Work out the finished part from the listing and answer in its coordinate system (mm). A direction names the side the tool comes from. Coordinates: 2 decimals unless noted, no trailing zeros. Order: outer loops, then holes, each group sorted by start corner. A loop starts at its lowest first (then second) coordinate and runs counter-clockwise, first axis right, second up.
```python
from build123d import *

# Parameters (mm, degrees)
F0_W      = 120.65
F0_H      = 120.65
F1_DEPTH  = 6.35
F2_W      = 12.7
F2_H      = 6.35
F3_DEPTH  = 6.351
F4_W      = 12.7
F4_H      = 6.35
F5_DEPTH  = 6.351
F6_W      = 6.35
F6_H      = 6.35
F7_DEPTH  = 6.351
F8_W      = 12.7
F8_H      = 6.35
F9_DEPTH  = 6.351
F10_W     = 12.7
F10_H     = 6.35
F11_DEPTH = 6.351
F12_W     = 6.35
F12_H     = 12.7
F13_DEPTH = 6.351
F14_W     = 6.35
F14_H     = 12.7
F15_DEPTH = 6.351
F16_W     = 6.35
F16_H     = 12.7
F17_DEPTH = 6.351
F18_W     = 12.7
F18_H     = 6.35
F19_DEPTH = 6.351
F20_W     = 12.7
F20_H     = 6.35
F20_W_2   = 6.35
F21_DEPTH = 6.351
F22_W     = 6.35
F22_H     = 12.7
F23_DEPTH = 6.351
F24_W     = 6.35
F24_H     = 12.7
F25_DEPTH = 6.351


with BuildPart() as f1:
    # F0 (on Right) → F1 (new body)
    with BuildSketch(Plane.YZ):
        Rectangle(F0_W, F0_H)
    extrude(amount=F1_DEPTH)

    # F2 (on face) → F3 (cut, through all)
    with BuildSketch(Plane(origin=(0, 0, 0), x_dir=(0, -1, 0), z_dir=(-1, 0, 0))):
        with Locations((53.975, 57.15)):
            Rectangle(F2_W, F2_H)
    extrude(amount=-F3_DEPTH, mode=Mode.SUBTRACT)

    # F4 (on face) → F5 (cut, through all)
    with BuildSketch(Plane(origin=(0, 0, 0), x_dir=(0, -1, 0), z_dir=(-1, 0, 0))):
        with Locations((28.575, 57.15)):
            Rectangle(F4_W, F4_H)
    extrude(amount=-F5_DEPTH, mode=Mode.SUBTRACT)

    # F6 (on face) → F7 (cut, through all)
    with BuildSketch(Plane(origin=(0, 0, 0), x_dir=(0, -1, 0), z_dir=(-1, 0, 0))):
        with Locations((0, 57.15)):
            Rectangle(F6_W, F6_H)
    extrude(amount=-F7_DEPTH, mode=Mode.SUBTRACT)

    # F8 (on face) → F9 (cut, through all)
    with BuildSketch(Plane(origin=(0, 0, 0), x_dir=(0, -1, 0), z_dir=(-1, 0, 0))):
        with Locations((-53.975, 57.15)):
            Rectangle(F8_W, F8_H)
    extrude(amount=-F9_DEPTH, mode=Mode.SUBTRACT)

    # F10 (on face) → F11 (cut, through all)
    with BuildSketch(Plane(origin=(0, 0, 0), x_dir=(0, -1, 0), z_dir=(-1, 0, 0))):
        with Locations((-28.575, 57.15)):
            Rectangle(F10_W, F10_H)
    extrude(amount=-F11_DEPTH, mode=Mode.SUBTRACT)

    # F12 (on face) → F13 (cut, through all)
    with BuildSketch(Plane(origin=(0, 0, 0), x_dir=(0, -1, 0), z_dir=(-1, 0, 0))):
        with Locations((-57.15, 34.925)):
            Rectangle(F12_W, F12_H)
    extrude(amount=-F13_DEPTH, mode=Mode.SUBTRACT)

    # F14 (on face) → F15 (cut, through all)
    with BuildSketch(Plane(origin=(0, 0, 0), x_dir=(0, -1, 0), z_dir=(-1, 0, 0))):
        with Locations((-57.15, 4.7625)):
            Rectangle(F14_W, F14_H)
    extrude(amount=-F15_DEPTH, mode=Mode.SUBTRACT)

    # F16 (on face) → F17 (cut, through all)
    with BuildSketch(Plane(origin=(0, 0, 0), x_dir=(0, -1, 0), z_dir=(-1, 0, 0))):
        with Locations((-57.15, -25.4)):
            Rectangle(F16_W, F16_H)
    extrude(amount=-F17_DEPTH, mode=Mode.SUBTRACT)

    # F18 (on face) → F19 (cut, through all)
    with BuildSketch(Plane(origin=(0, 0, 0), x_dir=(0, -1, 0), z_dir=(-1, 0, 0))):
        with Locations((-53.975, -57.15)):
            Rectangle(F18_W, F18_H)
        with Locations((53.975, -57.15)):
            Rectangle(F18_W, F18_H)
    extrude(amount=-F19_DEPTH, mode=Mode.SUBTRACT)

    # F20 (on face) → F21 (cut, through all)
    with BuildSketch(Plane(origin=(0, 0, 0), x_dir=(0, -1, 0), z_dir=(-1, 0, 0))):
        with Locations((-28.575, -57.15)):
            Rectangle(F20_W, F20_H)
        with Locations((0, -57.15)):
            Rectangle(F20_W_2, F20_H)
        with Locations((28.575, -57.15)):
            Rectangle(F20_W, F20_H)
    extrude(amount=-F21_DEPTH, mode=Mode.SUBTRACT)

    # F22 (on face) → F23 (cut, through all)
    with BuildSketch(Plane(origin=(0, 0, 0), x_dir=(0, -1, 0), z_dir=(-1, 0, 0))):
        with Locations((57.15, 34.925)):
            Rectangle(F22_W, F22_H)
        with Locations((57.15, 4.7625)):
            Rectangle(F22_W, F22_H)
    extrude(amount=-F23_DEPTH, mode=Mode.SUBTRACT)

    # F24 (on face) → F25 (cut, through all)
    with BuildSketch(Plane(origin=(0, 0, 0), x_dir=(0, -1, 0), z_dir=(-1, 0, 0))):
        with Locations((57.15, -25.4)):
            Rectangle(F24_W, F24_H)
    extrude(amount=-F25_DEPTH, mode=Mode.SUBTRACT)


solid = f1.part
```
1. Consider probe 1 along Z at (x, y) = (2, -52.5) (3 decimals). Determine where the line is inside the solid, lowest interval first.
2. The mould has two halves that part along Z. Classify faces 6 (the flat face through (3, 29, 53.975)), 7 (the flat face through (3, 60.325, -10)), 8 (the flat face through (3, 57, 41.275)): released by +Z, released by -Z, zero draft, split by the parting line, or undercut.
3. Flat-ended cylindrical pins translate along their axes: pin 1 (3 mm diameter, centred on x = 3.5, y = 57, fed in from -Z) (3 decimals); pin 2 (1 mm diameter, centred on x = 4, z = -26, fed in from -Y) (3 decimals); pin 3 (3 mm diameter, centred on x = 3, z = 34, fed in from +Y) (3 decimals). Find the tip coordinate at first contact, or state that the pin passes through.
4. The part is cut by section A-A (z = -26). Determine the outline of the cut face in (x, y) (3 decimals).
5. For faces 1 (the flat face through (3, 3.175, 57)), 2 (the flat face through (3, 34.925, -57)), 3 (the flat face through (3, -47.625, -57)), 4 (the flat face through (3, 57, 11.112)), 5 (the flat face through (3, -57, -31.75)), determine the directions among +Z, -Z, +X, -X, +Y, -Y from which every point of the face is accessible in a straight line to the end or side of a thin tool.
Worked out:
1. probe 1: z = -53.975 to 53.975
2. face 6: released by +Z
2. face 7: zero draft
2. face 8: undercut
3. pin 1: stops at z = -53.975
3. pin 2: stops at y = -53.975
3. pin 3: stops at y = 53.975
4. outline: (0, -53.975) - (6.35, -53.975) - (6.35, 53.975) - (0, 53.975) - close
5. face 1: +Z, +X, -X
5. face 2: -Z, +X, -X
5. face 3: -Z, +X, -X, -Y
5. face 4: +X, -X, +Y
5. face 5: +X, -X, -Y
